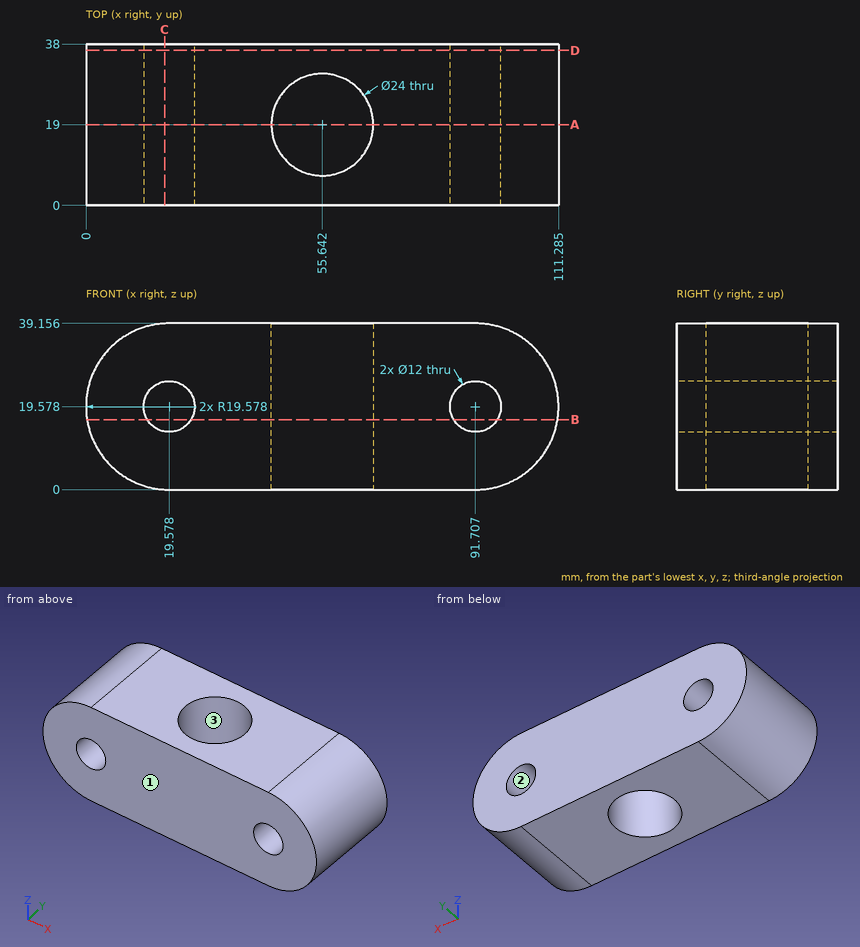
Geometry check sheet. Reference: drawing and pictorial views, mm from the part's lowest x, y, z. Round coordinates to 2 decimals unless told otherwise and drop trailing zeros. Write each loop counter-clockwise with the first axis right and the second up, starting at its lowest first coordinate (ties: lowest second). Pieces come first, ordered by that corner, then holes.
(1) Section check A-A (y = 19). Enter the section's corners in (x, z) (1 decimal), plus the area to 3 significant figures.
Returned:
outline: (19.6, 0) - (43.6, 0) - (43.6, 39.2) - (19.6, 39.2) arc R19.6 ccw to start; (67.6, 0) - (91.7, 0) arc R19.6 ccw to (91.7, 39.2) - (67.6, 39.2) - close; hole circle Ø12 at (19.6, 19.6); hole circle Ø12 at (91.7, 19.6)
area: 2,860 mm2
(2) Section check B-B (z = 16.5). Enter the section's corners in (x, y).
Returned:
outline: (0.24, 0) - (14.43, 0) - (14.43, 38) - (0.24, 38) - close; (24.73, 0) - (86.56, 0) - (86.56, 38) - (24.73, 38) - close; (96.86, 0) - (111.04, 0) - (111.04, 38) - (96.86, 38) - close; hole circle Ø24 at (55.64, 19)
(3) Section check C-C (x = 18.5). Enter the section's corners in (y, z) (1 decimal), plus the area to 3 significant figures.
Returned:
outline: (0, 0) - (38, 0) - (38, 13.7) - (0, 13.7) - close; (0, 25.5) - (38, 25.5) - (38, 39.1) - (0, 39.1) - close
area: 1,040 mm2
(4) Mould release check, pull along Y, two halves, no side actions. Record for the marked faces 1, 2 and 3: pulls with the +Y half, pulls with the -Y half, needs draft (parallel to the pull), parting line crosses it, or undercut.
Returned:
face 1: pulls with the -Y half
face 2: needs draft
face 3: undercut
(5) Depth check by flat-ended pin: pin 1 Ø5 at (y, z) = (15, 7) entering from -X; pin 2 Ø12 at (y, z) = (29, 24) entering from +X (1 decimal); pin 3 Ø6 at (y, z) = (33.5, 33) entering from -X (1 decimal). Enter the tip coordinate at first touch or a pass-through.
Returned:
pin 1: stops at x = 2.79
pin 2: stops at x = 111.3
pin 3: stops at x = 3
(6) Material ranges on line 1 (Y direction, x = 56, z = 29.5) (1 decimal); line 2 (Z direction, x = 92, y = 23.5) (1 decimal); line 3 (X direction, y = 31.5, z = 15) (1 decimal), recorded low to high.
Returned:
line 1: y = 0 to 7, 31 to 38
line 2: z = 0 to 13.6, 25.6 to 39.2
line 3: x = 0.5 to 15.7, 23.5 to 87.8, 95.6 to 110.7
(7) Section check D-D (y = 36.5). Enter the section's corners in (x, z) (1 decimal), plus the area to 3 significant figures.
Returned:
outline: (19.6, 0) - (91.7, 0) arc R19.6 ccw to (91.7, 39.2) - (19.6, 39.2) arc R19.6 ccw to start; hole circle Ø12 at (19.6, 19.6); hole circle Ø12 at (91.7, 19.6)
area: 3,800 mm2
